```python
from build123d import *

# Parameters (mm, degrees)
FILLET_1_R               = 0.2
CUT_EXTRUDE_2_REACH      = 50.223
PATTERN_CIRCULAR_1_COUNT = 5
CUT_EXTRUDE_3_REACH      = 50.223
SKETCH_8_R               = 4
CUT_EXTRUDE_4_REACH      = 50.223
SKETCH_9_R               = 2.1
PATTERN_CIRCULAR_2_COUNT = 5
CHAMFER_1_SIZE           = 2.2


with BuildPart() as part:
    # 草图2 → 旋转1 (revolve)
    with BuildSketch(Plane.XY, mode=Mode.PRIVATE) as revolve_1_sk:
        Polygon((0, 15.6), (0, -15.6), (26, -15.6), (26, -11), (24, -11), (24, -7.5), (25.2, -7.5), (24, -6.5), (24, 6.5), (25.2, 7.5), (24, 7.5), (24, 11), (26, 11), (26, 15.6), align=None)
    revolve(revolve_1_sk.sketch.rotate(Axis((0, 24.034054419, 0), (0, -1, 0)), 180), axis=Axis((0, 24.034054419, 0), (0, -1, 0)))

    # 圆角1
    fillet_1_edges = [part.edges().sort_by_distance(p)[0] for p in [
        (25.2, 7.5, 0),
        (25.2, -7.5, 0),
    ]]
    fillet(fillet_1_edges, radius=FILLET_1_R)

    # 草图6 → 切除-拉伸2 (cut, up to next)
    with BuildSketch(Plane.XZ.offset(15.6), mode=Mode.PRIVATE) as cut_extrude_2_sk1:
        with BuildLine():
            Line((9.090169944, -1.25227364), (17.376032265, 1.439966228))
            ThreePointArc((17.376032265, 1.439966228), (19.190312951, 1.140661306), (19.993406948, -0.513496449))
            ThreePointArc((19.993406948, -0.513496449), (19.021130326, -6.180339887), (16.476831637, -11.336402393))
            ThreePointArc((16.476831637, -11.336402393), (14.854825412, -12.202597321), (13.211114484, -11.378332658))
            Line((13.211114484, -11.378332658), (8.090169944, -4.329957177))
            ThreePointArc((8.090169944, -4.329957177), (7.8060909, -2.536352684), (9.090169944, -1.25227364))
        make_face()
    cut_extrude_2_tool1 = extrude(cut_extrude_2_sk1.sketch, amount=-CUT_EXTRUDE_2_REACH, mode=Mode.PRIVATE) & part.part
    cut_extrude_2 = cut_extrude_2_tool1.solids().sort_by_distance((14.482969, -15.6, -4.705802))[0]
    add(cut_extrude_2, mode=Mode.SUBTRACT)

    # 阵列(圆周)1: 切除-拉伸2 ×5 about axis
    pattern_circular_1_axis = Axis((0, 0, 0), (0, 1, 0))
    for i in range(1, PATTERN_CIRCULAR_1_COUNT):
        add(cut_extrude_2.rotate(pattern_circular_1_axis, i * 360 / PATTERN_CIRCULAR_1_COUNT), mode=Mode.SUBTRACT)

    # 草图8 → 切除-拉伸3 (cut, up to next)
    with BuildSketch(Plane(origin=(0, 15.6, 0), x_dir=(1, 0, 0), z_dir=(0, 1, 0)), mode=Mode.PRIVATE) as cut_extrude_3_sk1:
        with Locations(Location((0, 0, 0), (0, 0, 180))):
            Circle(SKETCH_8_R)
    cut_extrude_3_tool1 = extrude(cut_extrude_3_sk1.sketch, amount=-CUT_EXTRUDE_3_REACH, mode=Mode.PRIVATE) & part.part
    add(cut_extrude_3_tool1.solids().sort_by_distance((0, 15.6, 0))[0], mode=Mode.SUBTRACT)

    # 草图9 → 切除-拉伸4 (cut, up to next)
    with BuildSketch(Plane(origin=(0, 15.6, 0), x_dir=(1, 0, 0), z_dir=(0, 1, 0)), mode=Mode.PRIVATE) as cut_extrude_4_sk1:
        with Locations(Location((0, -15, 0), (0, 0, 180))):
            Circle(SKETCH_9_R)
    cut_extrude_4_tool1 = extrude(cut_extrude_4_sk1.sketch, amount=-CUT_EXTRUDE_4_REACH, mode=Mode.PRIVATE) & part.part
    cut_extrude_4 = cut_extrude_4_tool1.solids().sort_by_distance((0, 15.6, 15))[0]
    add(cut_extrude_4, mode=Mode.SUBTRACT)

    # 阵列(圆周)2: 切除-拉伸4 ×5 about axis
    pattern_circular_2_axis = Axis((0, 0, 0), (0, 1, 0))
    for i in range(1, PATTERN_CIRCULAR_2_COUNT):
        add(cut_extrude_4.rotate(pattern_circular_2_axis, i * 360 / PATTERN_CIRCULAR_2_COUNT), mode=Mode.SUBTRACT)

    # 倒角1
    chamfer_1_edges = [part.edges().sort_by_distance(p)[0] for p in [
        (26, -15.6, 0),
        (26, 15.6, 0),
    ]]
    chamfer(chamfer_1_edges, length=CHAMFER_1_SIZE)


solid = part.part
```
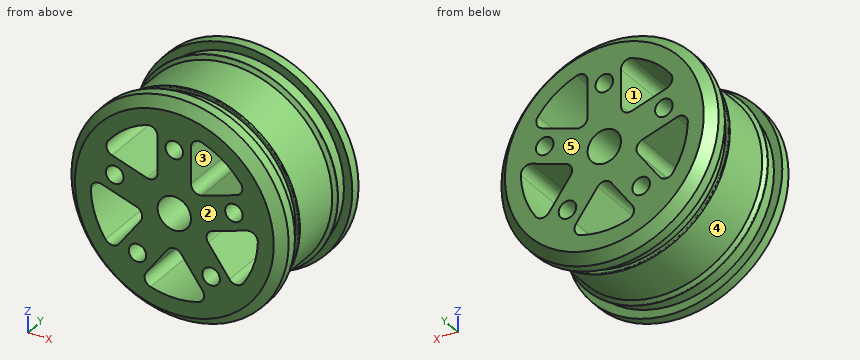
Source: CAD feature listing. Evaluate the final solid. Frame: model axes, mm. Face numbers are marked on the shaded views. A direction names the side the tool comes from. Round coordinates to 2 decimals unless told otherwise and drop trailing zeros.
1. Contact query for flat-ended pins moving along their axis: pin 1 (1 mm diameter, centred on y = 5, z = -17, fed in from -X); pin 2 (2 mm diameter, centred on x = -15.5, y = -0.5, fed in from +Z); pin 3 (6.5 mm diameter, centred on x = 14.27, z = 4.64, fed in from -Y); pin 4 (2.5 mm diameter, centred on y = 4, z = 12.5, fed in from -X). Output: stop coordinate, or through.
2. Mould query, pull axis Y, two halves, no side actions, for the marked faces 3, 4 and 5. Classes: released by +Y, released by -Y, zero draft, split by the parting line, or undercut.
3. Section query A-A on x = 0. Give the number of separate pieces and of enclosed holes in the cut face, and give its area (3 significant figures).
4. Ray query, L1, parallel to Z at x = -13, y = 5.5; L2, parallel to Z at x = 9, y = 4; L3, parallel to X at y = -1.5, z = -2. Return the intervals inside material, ascending.
5. Access query for the marked faces 1 and 2. Directions: +Z, -Z, +X, -X, +Y, -Y. A direction counts if a zero-diameter tool reaches every point of the face in a straight line with its end or side. Return the directions, or none.
Answers below:
1. pin 1: stops at x = -17.43
1. pin 2: stops at z = 19.12
1. pin 3: stops at y = -15.6
1. pin 4: stops at x = -21.2
2. face 3: zero draft
2. face 4: undercut
2. face 5: released by +Y
3. separate pieces: 4
3. enclosed holes: 0
3. area: 778 mm2
4. L1: z = -20.17 to -11.09, 0.02 to 2.96, 6.31 to 8.43, 15.2 to 20.17
4. L2: z = -22.25 to -14.23, -10.04 to -5.58, -1.28 to 7.13, 17.86 to 22.25
4. L3: x = -23.92 to -19.9, -8.07 to -3.46, 3.46 to 8.07, 19.9 to 23.92
5. face 1: +Y, -Y
5. face 2: +Z, -Z, +X, -X, -Y
